Autodesk Inventor part; units mm, degrees
ref_plane "YZ Plane" through (0, 0, 0) normal (1, 0, 0) x (0, 1, 0)
ref_plane "XZ Plane" through (0, 0, 0) normal (0, 1, 0) x (-1, 0, 0)
ref_plane "XY Plane" through (0, 0, 0) normal (0, 0, 1) x (1, 0, 0)
sketch "Szkic1" plane through (0, 0, 0) normal (0, 0, 1) x (1, 0, 0)
  line L0 (-10.3866, 5.557) -> (25.6134, 5.557)
  line L1 (25.6134, 5.557) -> (25.6134, -36.443)
  line L2 (25.6134, -36.443) -> (-10.3866, -36.443)
  line L3 (-10.3866, -36.443) -> (-10.3866, 5.557)
  point P0 (0, 0)
  point P1 (20.6134, -0.193)
  point P2 (20.6134, -30.693)
  point P3 (-5.3866, -0.193)
  point P4 (-5.3866, -30.693)
  dimension "d0" = 36
  dimension "d1" = 42
  dimension "d2" = 5
  dimension "d3" = 5
  dimension "d4" = 5
  dimension "d5" = 5
  dimension "d6" = 5.75
  dimension "d7" = 5.75
  dimension "d8" = 5.75
  dimension "d9" = 5.75
extrude "Wyciągnięcie proste1" add sketch "Szkic1" along normal blind 7.5
hole "Otwór1" at (20.6134, -0.193, 0) at (20.6134, -30.693, 0) at (-5.3866, -0.193, 0) at (-5.3866, -30.693, 0) direction (0, 0, 1) diameter 5 end through all
sketch "Szkic2" plane through (-10.3866, -36.443, 0) normal (0, -1, 0) x (1, 0, 0)
  line L0 (36, 0) -> (0, 0)
  line L1 (36, 0) -> (36, 7.5)
  line L2 (0, 7.5) -> (36, 7.5)
  line L3 (0, 0) -> (0, 7.5)
  line L4 (36, 7.5) -> (0, 7.5)
  circle A0 centre (18, 8.5) radius 5.05
  point P0 (10.3866, 0)
  dimension "d19" = 36
  dimension "d25" = 8.5
  dimension "d26" = 18
  dimension "d27" = 10.1
  dimension "d28" = 7.5
extrude "Wyciągnięcie proste2" cut sketch "Szkic2" against normal through all contours A0 L2 | L2 A0
fillet "Zaokrąglenie1" radius 1 4 edges at (-10.3866, -36.443, 3.75) (-10.3866, 5.557, 3.75) (25.6134, -36.443, 3.75) (25.6134, 5.557, 3.75)
properties part number "3DP_ABS_X_Axis_Linear_Shaft_Clamp_Top"
Could you check a few things on this model? Use its own coordinates, in mm. Coordinates: 2 decimals unless noted, no trailing zeros. Write each loop counter-clockwise with the first axis right and the second up, starting at its lowest first coordinate (ties: lowest second). Pieces come first, ordered by that corner, then holes. Notation, with made-up numbers: (3.5, 79) -> (18.5, 79) arc R20 cw to (18.5, 109) -> close; hole circle Ø7 at (-16, 37.5). An arc over 180 degrees is marked (long way). One line per question, with ' | ' between items. Start each with the question number.
1. If we section it at A-A (z = 5): Please give me the cut outline in (x, y).
2. If we section it at D-D (z = 1.25): Please give me the cut outline in (x, y), and give its area (3 significant figures).
3. If we section it at C-C (y = -9.5): Please give me the cut outline in (x, z).
4. Thinking about a two-plate mould opening in Y: for faces 1 (the face through (-2.946, -0.735, 3.802)), 2 (the face through (7, 5.557, 3)), 3 (the face through (23.054, -0.735, 3.802)), 4 (the face through (7, -15, 0)), which applies, pulls with the +Y half, pulls with the -Y half, needs draft (parallel to the pull), parting line crosses it, or undercut?
5. If we section it at B-B (x = -4): Please give me the cut outline in (y, z), and give its area (3 significant figures).
6. Please list where these lines run through material, in increasing order: line 1 along Y through (x, z) = (-6, 5.5); line 2 along X through (y, z) = (-2, 2); line 3 along X through (y, z) = (2, 2.5).
7. Will this pin go through, and if not, where does the flat tip stop? P1, Ø1.5, axis at x = 10, y = -20, coming from the +Z side.
Return value:
1) outline: (-10.39, -35.44) arc R1 ccw to (-9.39, -36.44) -> (3.97, -36.44) -> (3.97, 5.56) -> (-9.39, 5.56) arc R1 ccw to (-10.39, 4.56) -> close; (11.25, -36.44) -> (24.61, -36.44) arc R1 ccw to (25.61, -35.44) -> (25.61, 4.56) arc R1 ccw to (24.61, 5.56) -> (11.25, 5.56) -> close; hole circle Ø5 at (-5.39, -30.69); hole circle Ø5 at (-5.39, -0.19); hole circle Ø5 at (20.61, -30.69); hole circle Ø5 at (20.61, -0.19)
2) outline: (-10.39, -35.44) arc R1 ccw to (-9.39, -36.44) -> (24.61, -36.44) arc R1 ccw to (25.61, -35.44) -> (25.61, 4.56) arc R1 ccw to (24.61, 5.56) -> (-9.39, 5.56) arc R1 ccw to (-10.39, 4.56) -> close; hole circle Ø5 at (-5.39, -30.69); hole circle Ø5 at (-5.39, -0.19); hole circle Ø5 at (20.61, -30.69); hole circle Ø5 at (20.61, -0.19) | area: 1,430 mm²
3) outline: (-10.39, 0) -> (25.61, 0) -> (25.61, 7.5) -> (12.56, 7.5) arc R5.05 cw to (2.66, 7.5) -> (-10.39, 7.5) -> close
4) face 1: undercut | face 2: pulls with the +Y half | face 3: undercut | face 4: needs draft
5) outline: (-36.44, 0) -> (-32.77, 0) -> (-32.77, 7.5) -> (-36.44, 7.5) -> close; (-28.61, 0) -> (-2.27, 0) -> (-2.27, 7.5) -> (-28.61, 7.5) -> close; (1.89, 0) -> (5.56, 0) -> (5.56, 7.5) -> (1.89, 7.5) -> close | area: 253 mm²
6) line 1: y = -36.44 to -33.12, -28.27 to -2.62, 2.23 to 5.56 | line 2: x = -10.39 to -7.11, -3.66 to 18.89, 22.34 to 25.61 | line 3: x = -10.39 to -6.59, -4.19 to 19.41, 21.81 to 25.61
7) P1: stops at z = 4.54
